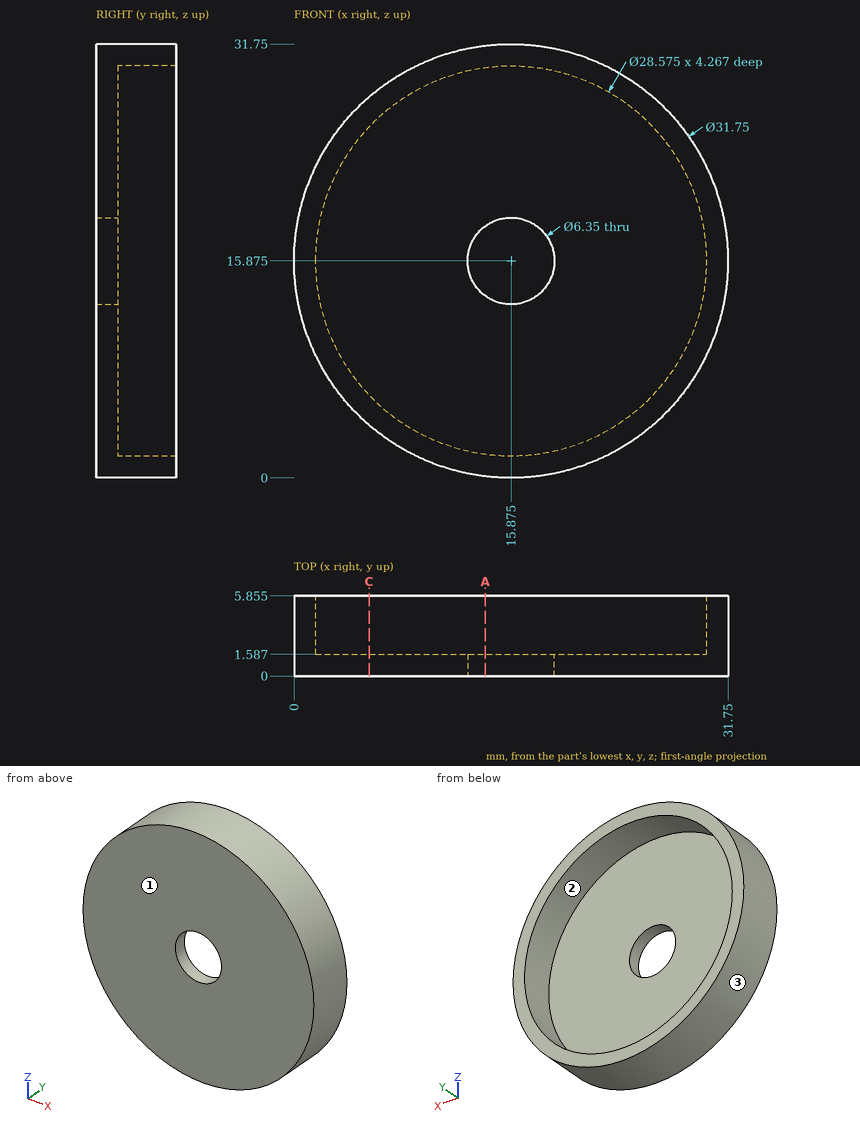
Could you check a few things on this drawing? It's one solid part, dimensions in mm from its lowest x, y, z. Give positions to 0.01 mm unless a question says otherwise; leave off trailing zeros. Order: outer loops, then holes, each group sorted by start corner. A loop starts at its lowest first (then second) coordinate and runs counter-clockwise, first axis right, second up. Notation, with made-up numbers: (1.25, -28) -> (27.25, -28) arc R19 cw to (27.25, 6) -> close; hole circle Ø5 at (81.25, 64.5). An arc over 180 degrees is marked (long way). Use CSV: the item, a comma, the result in double quotes. Start each with the question number.
Item 1: Thinking about a two-plate mould opening in X: for the marked faces 1, 2 and 3, which applies, pulls with the +X half, pulls with the -X half, needs draft (parallel to the pull), parting line crosses it, or undercut?
Item 2: I'm going to push flat-ended pins straight in: P1, Ø10, axis at x = 27, z = 23, coming from the -Y side; P2, Ø3, axis at x = 10, z = 5, coming from the +Y side. Where does each tip first touch, or does it pass through?
Item 3: Suppose I cut it at C-C (x = 5.5). List the corners of the cut face in (y, z) for me (1 decimal).
Item 4: Suppose I cut it at A-A (x = 14). List the corners of the cut face in (y, z) for me (1 decimal).
Item 5: If I drill on probe 1 along Y at (x, z) = (2, 17); probe 2 along X at (y, z) = (3.3, 11.5) (1 decimal); probe 3 along X at (y, z) = (3.35, 8.5) (1 decimal), over which ranges is the centre line in solid material (lowest first)? Write a range as [from, to].
Answer block:
1,face 1,"needs draft"
1,face 2,"undercut"
1,face 3,"parting line crosses it"
2,P1,"stops at y = 0"
2,P2,"stops at y = 1.59"
3,outline,"(0, 3.9) -> (5.9, 3.9) -> (5.9, 6.1) -> (1.6, 6.1) -> (1.6, 25.7) -> (5.9, 25.7) -> (5.9, 27.9) -> (0, 27.9) -> close"
4,outline,"(0, 0.1) -> (5.9, 0.1) -> (5.9, 1.7) -> (1.6, 1.7) -> (1.6, 13.3) -> (0, 13.3) -> close; (0, 18.4) -> (1.6, 18.4) -> (1.6, 30) -> (5.9, 30) -> (5.9, 31.6) -> (0, 31.6) -> close"
5,probe 1,"y = [0, 1.59]"
5,probe 2,"x = [0.6, 2.3], [29.5, 31.1]"
5,probe 3,"x = [1.8, 3.6], [28.1, 29.9]"
